from build123d import *

# Parameters (mm, degrees)
SKETCH1_W               = 150
SKETCH1_H               = 300
BOSS_EXTRUDE1_DEPTH     = 10
FLANGE_SLIT_W           = 26
FLANGE_SLIT_H           = 2.2
FLANGE_SLOT_DEPTH       = 8
SKETCH3_W               = 7.5
SKETCH3_H               = 65
SKETCH6_W               = 57.250839866
SKETCH6_H               = 300
CUT_EXTRUDE2_DEPTH      = 169.002976164
SKETCH7_W               = 8.586676089
SKETCH7_H               = 4.428918394
CUT_EXTRUDE3_DEPTH      = 169.002976164
CUT_EXTRUDE3_DEPTH_BACK = 169.002976164
SKETCH15_W              = 274.383047756
SKETCH15_H              = 92.749160134


with BuildPart() as part:
    # Sketch1 → Boss-Extrude1 (new body)
    with BuildSketch(Plane(origin=(0, 0, 0), x_dir=(0, 1, 0), z_dir=(0, 0, 1))):
        Rectangle(SKETCH1_W, SKETCH1_H)
    extrude(amount=BOSS_EXTRUDE1_DEPTH)

    # flange slit → Flange Slot (cut)
    with BuildSketch(Plane.XY.offset(10)):
        with Locations((-137.383047756, -69.471081606)):
            Rectangle(FLANGE_SLIT_W, FLANGE_SLIT_H)
    extrude(amount=-FLANGE_SLOT_DEPTH, mode=Mode.SUBTRACT)

    # Sketch3 → Syringe Body Slot (revolve, cut)
    with BuildSketch(Plane.XY.offset(10)):
        with Locations((-140.941523878, -35.871081606)):
            Rectangle(SKETCH3_W, SKETCH3_H)
    revolve(axis=Axis((-137.191523878, 75, 10), (0, -1, 0)), mode=Mode.SUBTRACT)

    # Sketch6 → Cut-Extrude2 (cut, through all)
    with BuildSketch(Plane(origin=(0, 0, 10), x_dir=(0, -1, 0), z_dir=(0, 0, 1))):
        with Locations((-46.374580067, 0)):
            Rectangle(SKETCH6_W, SKETCH6_H)
    extrude(amount=-CUT_EXTRUDE2_DEPTH, mode=Mode.SUBTRACT)

    # Sketch7 → Plunger Slot (revolve, cut)
    with BuildSketch(Plane.XY.offset(10)):
        with Locations((-141.484861922, -72.785540803)):
            Rectangle(SKETCH7_W, SKETCH7_H)
    revolve(axis=Axis((-137.191523878, -70.571081606, 10), (0, -1, 0)), mode=Mode.SUBTRACT)

    # Sketch8 → Cut-Revolve1 (revolve, cut)
    with BuildSketch(Plane.XY.offset(10)):
        Polygon((-137.191523878, -3.371081606), (-141.791523878, -3.371081606), (-141.791523878, 7.236534378), (-139.709650935, 7.236534378), (-139.709650935, 17.749160134), (-137.191523878, 17.749160134), (-137.191523878, 4.628918394), align=None)
    revolve(axis=Axis((-137.191523878, -3.371081606, 10), (0, 1, 0)), mode=Mode.SUBTRACT)

    # Sketch15 → Cut-Extrude3 (cut, two sides: drawn at the far end of the back side and taken through both)
    with BuildSketch(Plane.XY.offset(10).offset(-CUT_EXTRUDE3_DEPTH_BACK)):
        with Locations((12.808476122, -28.625419933)):
            Rectangle(SKETCH15_W, SKETCH15_H)
    extrude(amount=CUT_EXTRUDE3_DEPTH + CUT_EXTRUDE3_DEPTH_BACK, mode=Mode.SUBTRACT)


solid = part.part
Check sheet for the modelled part. Datum: model origin and axes. Units: mm. A direction names the side the tool comes from. Coordinates: 2 decimals unless noted, no trailing zeros. Write each loop counter-clockwise with the first axis right and the second up, starting at its lowest first coordinate (ties: lowest second). Pieces come first, ordered by that corner, then holes.
Item 1: Mould release check, pull along Y, two halves, no side actions. Record for faces 1 (the face through (-134.2, -75, 1.6)), 2 (the face through (-124.383, -29, 5)), 3 (the face through (-127, -70.571, 5)): released by +Y, released by -Y, zero draft, split by the parting line, or undercut.
Numbers:
face 1: released by -Y
face 2: zero draft
face 3: undercut
Item 2: Cross-section at A-A on z = 4. Record the boundary of the cut face in (x, y), then the cut area to 3 significant figures.
Numbers:
outline: (-150, -75) - (-143.33, -75) - (-143.33, -70.57) - (-150, -70.57) - close; (-150, -68.37) - (-141.69, -68.37) - (-141.69, -3.37) - (-132.69, -3.37) - (-132.69, -68.37) - (-124.38, -68.37) - (-124.38, 17.75) - (-150, 17.75) - close; (-131.05, -75) - (-124.38, -75) - (-124.38, -70.57) - (-131.05, -70.57) - close
area: 1,680 mm2
Item 3: Scan lines: probe 1 along Y at (x, z) = (-147.75, 6.25); probe 2 along X at (y, z) = (-60, 9.5); probe 3 along Y at (x, z) = (-132.5, 5.25). Record each from-to range of solid material in increasing order.
Numbers:
probe 1: y = -75 to -70.57, -68.37 to 17.75
probe 2: x = -150 to -144.67, -129.71 to -124.38
probe 3: y = -3.37 to 17.75
Item 4: Cross-section at D-D on z = 8.5. Record the boundary of the cut face in (x, y), then the cut area to 3 significant figures.
Numbers:
outline: (-150, -75) - (-145.65, -75) - (-145.65, -70.57) - (-150, -70.57) - close; (-150, -68.37) - (-144.54, -68.37) - (-144.54, -3.37) - (-141.54, -3.37) - (-141.54, 7.24) - (-139.21, 7.24) - (-139.21, 17.75) - (-150, 17.75) - close; (-135.17, 7.24) - (-132.84, 7.24) - (-132.84, -3.37) - (-129.84, -3.37) - (-129.84, -68.37) - (-124.38, -68.37) - (-124.38, 17.75) - (-135.17, 17.75) - close; (-128.74, -75) - (-124.38, -75) - (-124.38, -70.57) - (-128.74, -70.57) - close
area: 1,150 mm2
Item 5: Depth check by flat-ended pin: pin 1 Ø1.1 at (x, y) = (-143, -69.5) entering from +Z; pin 2 Ø5 at (x, y) = (-135.5, -37.5) entering from +Z; pin 3 Ø5 at (x, z) = (-135.5, 8.5) entering from -Y. Enter the tip coordinate at first touch or a pass-through.
Numbers:
pin 1: stops at z = 2
pin 2: stops at z = 3.78
pin 3: stops at y = -3.37
Item 6: Access from +Z, -Z, +X, -X, +Y, -Y to the whole of each face (thin tool, end or side, straight path). Record for faces 4 (the face through (-137, -69, 2)), 5 (the face through (-137.1, 2, 5.4)), 6 (the face through (-137, -29, 0)).
Numbers:
face 4: +Z, +X, -X
face 5: +Z, -Y
face 6: -Z, +X, -X, +Y, -Y
Item 7: Cross-section at B-B on y = 4. Record the boundary of the cut face in (x, z).
Numbers:
outline: (-150, 0) - (-124.38, 0) - (-124.38, 10) - (-132.59, 10) arc R4.6 cw to (-141.79, 10) - (-150, 10) - close
Item 8: Cross-section at C-C on x = -126. Record the boundary of the cut face in (y, z), then the cut area to 3 significant figures.
Numbers:
outline: (-75, 0) - (17.75, 0) - (17.75, 10) - (-68.37, 10) - (-68.37, 2) - (-70.57, 2) - (-70.57, 10) - (-75, 10) - close
area: 910 mm2
